Model file for the job. Use its own axes, mm. Round coordinates to 2 decimals unless told otherwise and drop trailing zeros. Loops run counter-clockwise (first coordinate to the right, second up) from the corner with the lowest first, then second, coordinate; pieces in that order, holes last. Notation, with made-up numbers: (24.25, -6.75) - (54.25, -6.75) arc R19 ccw to (54.25, 20.25) - close; hole circle Ø3 at (-21, -28). An arc over 180 degrees is marked (long way). Use one line per item in the form item = value.
from build123d import *

# Parameters (mm, degrees)
ESQUISSE1_W             = 19
ESQUISSE1_H             = 35.6
BOSS_EXTRU_1_DEPTH      = 1
ESQUISSE2_W             = 17
ESQUISSE2_H             = 34.5
BOSS_EXTRU_2_DEPTH      = 2.2
ESQUISSE3_R             = 0.5
ENL_V_MAT_EXTRU_1_DEPTH = 0.2
ESQUISSE4_R             = 0.75
ENL_V_MAT_EXTRU_2_DEPTH = 2


with BuildPart() as part:
    # Esquisse1 → Boss.-Extru.1 (new body)
    with BuildSketch(Plane(origin=(0, 0, 0), x_dir=(1, 0, 0), z_dir=(0, 1, 0))):
        with Locations((9.5, 17.8)):
            Rectangle(ESQUISSE1_W, ESQUISSE1_H)
    extrude(amount=BOSS_EXTRU_1_DEPTH)

    # Esquisse2 → Boss.-Extru.2 (add)
    with BuildSketch(Plane(origin=(0, 1, 0), x_dir=(1, 0, 0), z_dir=(0, 1, 0))):
        with Locations((9.5, 18.25)):
            Rectangle(ESQUISSE2_W, ESQUISSE2_H)
    extrude(amount=BOSS_EXTRU_2_DEPTH)

    # Esquisse3 → Enlèv. mat.-Extru.1 (cut)
    with BuildSketch(Plane(origin=(0, 3.2, 0), x_dir=(1, 0, 0), z_dir=(0, 1, 0))):
        with Locations((6, 6)):
            Circle(ESQUISSE3_R)
        with Locations((11, 6)):
            Circle(ESQUISSE3_R)
        with Locations((8.5, 8.5)):
            Circle(ESQUISSE3_R)
        with Locations((13.5, 8.5)):
            Circle(ESQUISSE3_R)
        with Locations((11, 11)):
            Circle(ESQUISSE3_R)
        with Locations((8.5, 13.5)):
            Circle(ESQUISSE3_R)
        with Locations((13.5, 13.5)):
            Circle(ESQUISSE3_R)
        with Locations((11, 16)):
            Circle(ESQUISSE3_R)
        with Locations((8.5, 18.5)):
            Circle(ESQUISSE3_R)
        with Locations((13.5, 18.5)):
            Circle(ESQUISSE3_R)
        with Locations((11, 21)):
            Circle(ESQUISSE3_R)
        with Locations((8.5, 23.5)):
            Circle(ESQUISSE3_R)
        with Locations((13.5, 23.5)):
            Circle(ESQUISSE3_R)
        with Locations((11, 26)):
            Circle(ESQUISSE3_R)
        with Locations((6, 11)):
            Circle(ESQUISSE3_R)
        with Locations((6, 16)):
            Circle(ESQUISSE3_R)
        with Locations((6, 21)):
            Circle(ESQUISSE3_R)
        with Locations((6, 26)):
            Circle(ESQUISSE3_R)
    extrude(amount=-ENL_V_MAT_EXTRU_1_DEPTH, mode=Mode.SUBTRACT)

    # Esquisse4 → Enlèv. mat.-Extru.2 (cut, through all)
    with BuildSketch(Plane(origin=(0, 1, 0), x_dir=(1, 0, 0), z_dir=(0, 1, 0))):
        with Locations((2.6, 0)):
            Circle(ESQUISSE4_R)
        with Locations((7.2, 0)):
            Circle(ESQUISSE4_R)
        with Locations((11.8, 0)):
            Circle(ESQUISSE4_R)
        with Locations((16.4, 0)):
            Circle(ESQUISSE4_R)
        with Locations((0, 4.45)):
            Circle(ESQUISSE4_R)
        with Locations((0, 8.9)):
            Circle(ESQUISSE4_R)
        with Locations((0, 13.35)):
            Circle(ESQUISSE4_R)
        with Locations((0, 17.8)):
            Circle(ESQUISSE4_R)
        with Locations((0, 22.25)):
            Circle(ESQUISSE4_R)
        with Locations((0, 26.7)):
            Circle(ESQUISSE4_R)
        with Locations((0, 31.15)):
            Circle(ESQUISSE4_R)
        with Locations((19, 4.45)):
            Circle(ESQUISSE4_R)
        with Locations((19, 8.9)):
            Circle(ESQUISSE4_R)
        with Locations((19, 13.35)):
            Circle(ESQUISSE4_R)
        with Locations((19, 17.8)):
            Circle(ESQUISSE4_R)
        with Locations((19, 22.25)):
            Circle(ESQUISSE4_R)
        with Locations((19, 26.7)):
            Circle(ESQUISSE4_R)
        with Locations((19, 31.15)):
            Circle(ESQUISSE4_R)
    extrude(amount=-ENL_V_MAT_EXTRU_2_DEPTH, mode=Mode.SUBTRACT)


solid = part.part
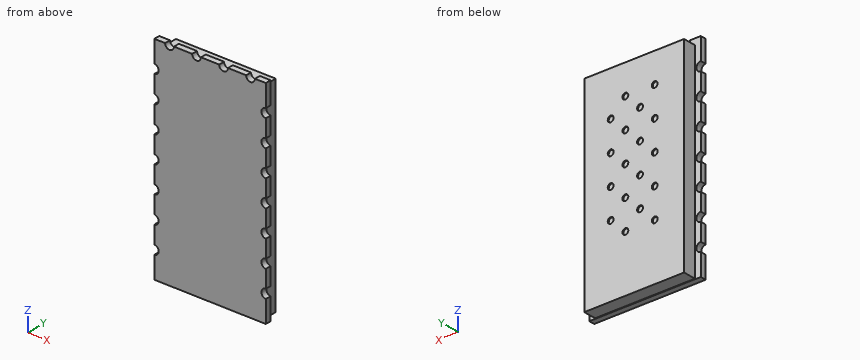
1. Wall check: probe 1 along X at (y, z) = (3.1, -8.5); probe 2 along X at (y, z) = (3.1, -26); probe 3 along Z at (x, y) = (11, 3.15). Give the ranges that are in metal, low to high.
Geometry check:
probe_1 = 1 to 8, 9 to 13, 14 to 18
probe_2 = 1 to 5.5, 6.5 to 10.5, 11.5 to 18
probe_3 = -35.5 to -26.5, -25.5 to -21.5, -20.5 to -16.5, -15.5 to -11.5, -10.5 to -6.5, -5.5 to -1
2. Cut at A-A, the plane z = -4.45. Give the cut face in (x, y).
Geometry check:
outline = (0.75, 0) - (18.25, 0) - (18.25, 1) - (18, 1) - (18, 3.2) - (1, 3.2) - (1, 1) - (0.75, 1) - close
3. Flat gauge pins, fed straight in: pin 1 (0.8 mm diameter, centred on x = 11, z = -16, fed in from +Y); pin 2 (0.7 mm diameter, centred on x = 6, y = 2.5, fed in from -Z); pin 3 (0.7 mm diameter, centred on y = 2, z = -21.5, fed in from +X). Where does each tip first touch, or does it go through?
Geometry check:
pin_1 = 3
pin_2 = -35.5
pin_3 = 18
4. Cut at C-C, the plane y = 1.9. Give the cut face in (x, z), plus the area to 4 significant figures.
Geometry check:
outline = (1, -35.5) - (18, -35.5) - (18, -1) - (1, -1) - close
area = 586.5 mm^2
5. Cut at B-B, the plane x = 15.25. Give the cut face in (y, z), plus the area to 4 significant figures.
Geometry check:
outline = (0, -35.6) - (1, -35.6) - (1, -35.5) - (3.2, -35.5) - (3.2, -1) - (1, -1) - (1, 0) - (0, 0) - close
area = 111.5 mm^2
6. Cut at D-D, the plane z = -11. Give the cut face in (x, y).
Geometry check:
outline = (0, 0) - (19, 0) - (19, 1) - (18, 1) - (18, 3.2) - (11.5, 3.2) - (11.5, 3) - (10.5, 3) - (10.5, 3.2) - (6.5, 3.2) - (6.5, 3) - (5.5, 3) - (5.5, 3.2) - (1, 3.2) - (1, 1) - (0, 1) - close
